Part print with two shaded views. Sizes in mm from the minimum x, y, z corner. A direction names the side the tool comes from. Give positions to 0.01 mm unless a question says otherwise; leave off trailing zeros. Order: outer loops, then holes, each group sorted by start corner. A loop starts at its lowest first (then second) coordinate and runs counter-clockwise, first axis right, second up. Notation, with made-up numbers: M -35.5,-3.75 L 3.5,-3.75 A22 ccw 3.5,29.25 Z; hole C -22,-37.5 d11. An arc over 180 degrees is marked long. Answer as CSV lines item,"result".
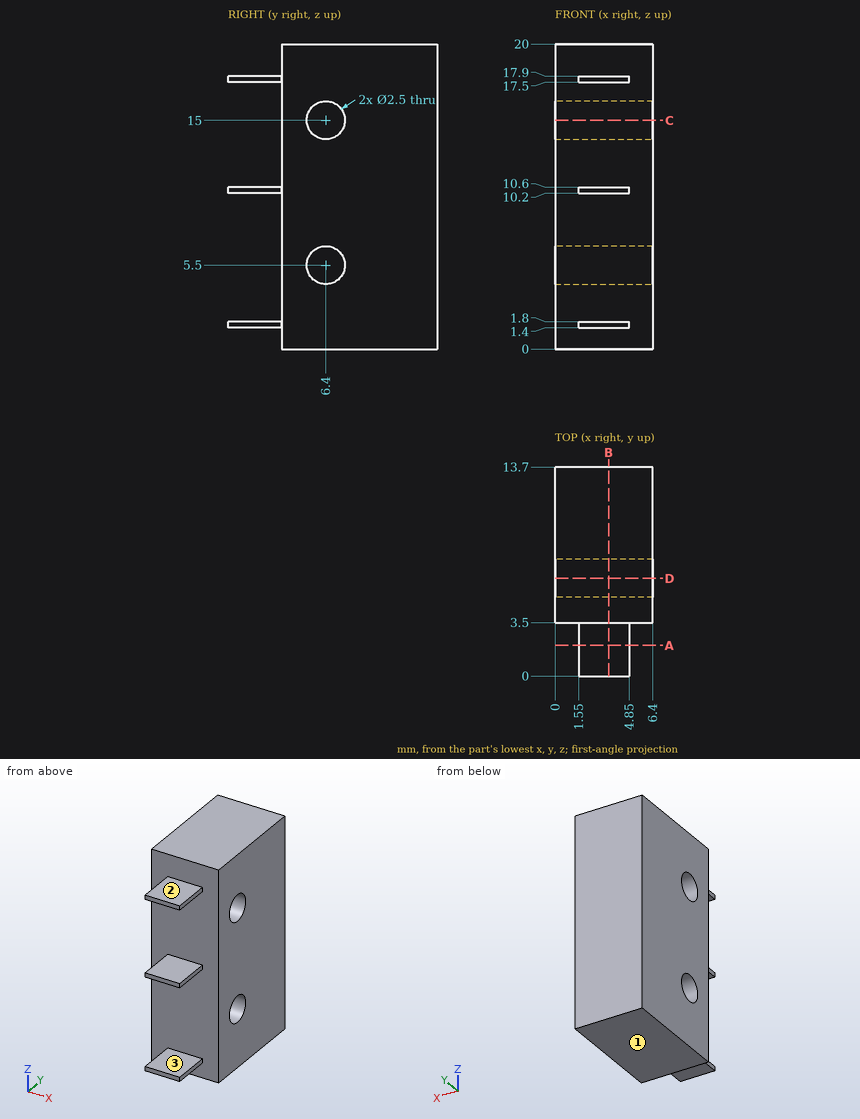
Item 1: Probe line 1 along Z through (x, y) = (1.5, 6.4); line 2 along Z through (x, y) = (4.5, 3); line 3 along Y through (x, z) = (4, 15). List the from-to ranges inside material, lowest first. Write a range as from..to.
Geometry says:
line 1,"z = 0..4.25, 6.75..13.75, 16.25..20"
line 2,"z = 1.4..1.8, 10.2..10.6, 17.5..17.9"
line 3,"y = 3.5..5.15, 7.65..13.7"
Item 2: Band-saw the part on D-D (y = 6.4). Give the cut face in (x, z), and give its area (3 significant figures).
Geometry says:
outline,"M 0,0 L 6.4,0 L 6.4,4.25 L 0,4.25 Z; M 0,6.75 L 6.4,6.75 L 6.4,13.75 L 0,13.75 Z; M 0,16.25 L 6.4,16.25 L 6.4,20 L 0,20 Z"
area,"96.0 mm2"
Item 3: Band-saw the part on C-C (z = 15). Give the cut face in (x, y).
Geometry says:
outline,"M 0,3.5 L 6.4,3.5 L 6.4,5.15 L 0,5.15 Z; M 0,7.65 L 6.4,7.65 L 6.4,13.7 L 0,13.7 Z"
Item 4: Band-saw the part on B-B (x = 3.5). Give the cut face in (y, z).
Geometry says:
outline,"M 0,1.4 L 3.5,1.4 L 3.5,0 L 13.7,0 L 13.7,20 L 3.5,20 L 3.5,17.9 L 0,17.9 L 0,17.5 L 3.5,17.5 L 3.5,10.6 L 0,10.6 L 0,10.2 L 3.5,10.2 L 3.5,1.8 L 0,1.8 Z; hole C 6.4,5.5 d2.5; hole C 6.4,15 d2.5"
Item 5: Drop flat-ended pins along their axis: pin 1 (1.6 mm diameter, centred on x = 4, y = 1, fed in from -Z); pin 2 (3.5 mm diameter, centred on x = 3, y = 1.5, fed in from +Z). Give the stop position or say it passes through.
Geometry says:
pin 1,"stops at z = 1.4"
pin 2,"stops at z = 17.9"
Item 6: 3-axis set-ups, long thin cutter, end or side, ignore diameter. For the marked faces 1, 2 and 3: which of +Z, -Z, +X, -X, +Y, -Y reach the whole face in a straight line?
Geometry says:
face 1,"-Z, +X, -X, +Y, -Y"
face 2,"+Z, +X, -X, -Y"
face 3,"+X, -X, -Y"
Item 7: Band-saw the part on A-A (y = 2). Give the cut face in (x, z).
Geometry says:
outline,"M 1.55,1.4 L 4.85,1.4 L 4.85,1.8 L 1.55,1.8 Z; M 1.55,10.2 L 4.85,10.2 L 4.85,10.6 L 1.55,10.6 Z; M 1.55,17.5 L 4.85,17.5 L 4.85,17.9 L 1.55,17.9 Z"
